from build123d import *

# Parameters (mm, degrees)
BOTTOMSKETCH_W               = 30
BOTTOMSKETCH_H               = 30
BOTTOMEXTRUSION_DEPTH        = 3
HOLESKETCH_W                 = 10.3
HOLESKETCH_H                 = 10.3
HOLEEXTRUSION_DEPTH          = 2
LATERALWIRESKETCH_W          = 4.7
LATERALWIRESKETCH_H          = 2
LATERALWIREEXTRUSION_DEPTH   = 2
WIRERESEVOIRSKETCH_W         = 2
WIRERESEVOIRSKETCH_H         = 21.5
WIRERESERVOIREXTRUSION_DEPTH = 2


with BuildPart() as part:
    # bottomSketch → bottomExtrusion (new body)
    with BuildSketch(Plane(origin=(0, 0, 0), x_dir=(1, 0, 0), z_dir=(0, 1, 0))):
        Rectangle(BOTTOMSKETCH_W, BOTTOMSKETCH_H)
    extrude(amount=BOTTOMEXTRUSION_DEPTH)

    # holeSketch → holeExtrusion (cut)
    with BuildSketch(Plane(origin=(0, 3, 0), x_dir=(1, 0, 0), z_dir=(0, 1, 0))):
        with Locations((-7.5, 7.5)):
            Rectangle(HOLESKETCH_W, HOLESKETCH_H)
        with Locations((-7.5, -7.5)):
            Rectangle(HOLESKETCH_W, HOLESKETCH_H)
        with Locations((7.5, 7.5)):
            Rectangle(HOLESKETCH_W, HOLESKETCH_H)
        with Locations((7.5, -7.5)):
            Rectangle(HOLESKETCH_W, HOLESKETCH_H)
    extrude(amount=-HOLEEXTRUSION_DEPTH, mode=Mode.SUBTRACT)

    # lateralWireSketch → lateralWireExtrusion (cut)
    with BuildSketch(Plane(origin=(0, 3, 0), x_dir=(1, 0, 0), z_dir=(0, 1, 0))):
        with Locations((0, -7.5)):
            Rectangle(LATERALWIRESKETCH_W, LATERALWIRESKETCH_H)
        with Locations((0, 7.5)):
            Rectangle(LATERALWIRESKETCH_W, LATERALWIRESKETCH_H)
    extrude(amount=-LATERALWIREEXTRUSION_DEPTH, mode=Mode.SUBTRACT)

    # wireResevoirSketch → wireReservoirExtrusion (cut)
    with BuildSketch(Plane(origin=(0, 3, 0), x_dir=(1, 0, 0), z_dir=(0, 1, 0))):
        with Locations((0, -4.25)):
            Rectangle(WIRERESEVOIRSKETCH_W, WIRERESEVOIRSKETCH_H)
    extrude(amount=-WIRERESERVOIREXTRUSION_DEPTH, mode=Mode.SUBTRACT)


solid = part.part
Could you check a few things on this model? Use its own coordinates, in mm. Coordinates: 2 decimals unless noted, no trailing zeros. Write each loop counter-clockwise with the first axis right and the second up, starting at its lowest first coordinate (ties: lowest second). Pieces come first, ordered by that corner, then holes. Notation, with made-up numbers: (46.25, -37) - (77.25, -37) arc R17 cw to (77.25, -8) - close; hole circle Ø9 at (57, -22.5). An arc over 180 degrees is marked (long way). Put each result on its own line as item: value. Start each with the question number.
Q1. Please list where these lines run through material, in increasing order: L1, parallel to Z at x = -2, y = 2.45; L2, parallel to Z at x = 12, y = 2.3; L3, parallel to X at y = 1.15, z = -3.25.
Q2. I want a section at C-C on z = -7.5. Write out the boundary of the cut face in (x, y), plus the area to 3 significant figures.
Q3. I want a section at B-B on x = -12. Write out the boundary of the cut face in (y, z), plus the area to 3 significant figures.
Q4. I'm going to push a flat-ended pin straight in: P1, Ø6, axis at x = 5, z = -5, coming from the -Y side. Where does the tip first touch, or does it pass through?
Q5. I want a section at A-A on z = -3.5. Write out the boundary of the cut face in (x, y), plus the area to 3 significant figures.
Q6. Thinking about a two-plate mould opening in Z: for faces 1 (the flat face through (0, 0, 0)), 2 (the flat face through (-0.2, 0.8, 15)), 3 (the flat face through (-2.35, 2, -11)), which applies, pulls with the +Z half, pulls with the -Z half, needs draft (parallel to the pull), parting line crosses it, or undercut?
Q7. I want a section at D-D on x = 1.5. Write out the boundary of the cut face in (y, z).
Checks:
1. L1: -15 to -8.5, -6.5 to 6.5, 8.5 to 15
1. L2: -15 to -12.65, -2.35 to 2.35, 12.65 to 15
1. L3: -15 to -12.65, -2.35 to -1, 1 to 2.35, 12.65 to 15
2. outline: (-15, 0) - (15, 0) - (15, 3) - (12.65, 3) - (12.65, 1) - (-12.65, 1) - (-12.65, 3) - (-15, 3) - close
2. area: 39.4 mm²
3. outline: (0, -15) - (3, -15) - (3, -12.65) - (1, -12.65) - (1, -2.35) - (3, -2.35) - (3, 2.35) - (1, 2.35) - (1, 12.65) - (3, 12.65) - (3, 15) - (0, 15) - close
3. area: 48.8 mm²
4. P1: y = 0
5. outline: (-15, 0) - (15, 0) - (15, 3) - (12.65, 3) - (12.65, 1) - (2.35, 1) - (2.35, 3) - (1, 3) - (1, 1) - (-1, 1) - (-1, 3) - (-2.35, 3) - (-2.35, 1) - (-12.65, 1) - (-12.65, 3) - (-15, 3) - close
5. area: 44.8 mm²
6. face 1: needs draft
6. face 2: pulls with the +Z half
6. face 3: undercut
7. outline: (0, -15) - (3, -15) - (3, -8.5) - (1, -8.5) - (1, -6.5) - (3, -6.5) - (3, 6.5) - (1, 6.5) - (1, 8.5) - (3, 8.5) - (3, 15) - (0, 15) - close
